Drawing for the job (mm, zero at the part's lowest x, y, z). A direction names the side the tool comes from. Round coordinates to 2 decimals unless told otherwise and drop trailing zeros. Write each loop counter-clockwise with the first axis right and the second up, starting at its lowest first coordinate (ties: lowest second). Pieces come first, ordered by that corner, then holes. Notation, with made-up numbers: (-19.5, 58) - (-5.5, 58) arc R30 cw to (-5.5, 87) - close; hole circle Ø7 at (-39.5, 34.25). An arc over 180 degrees is marked (long way). Answer in a Markdown table with one row per item.
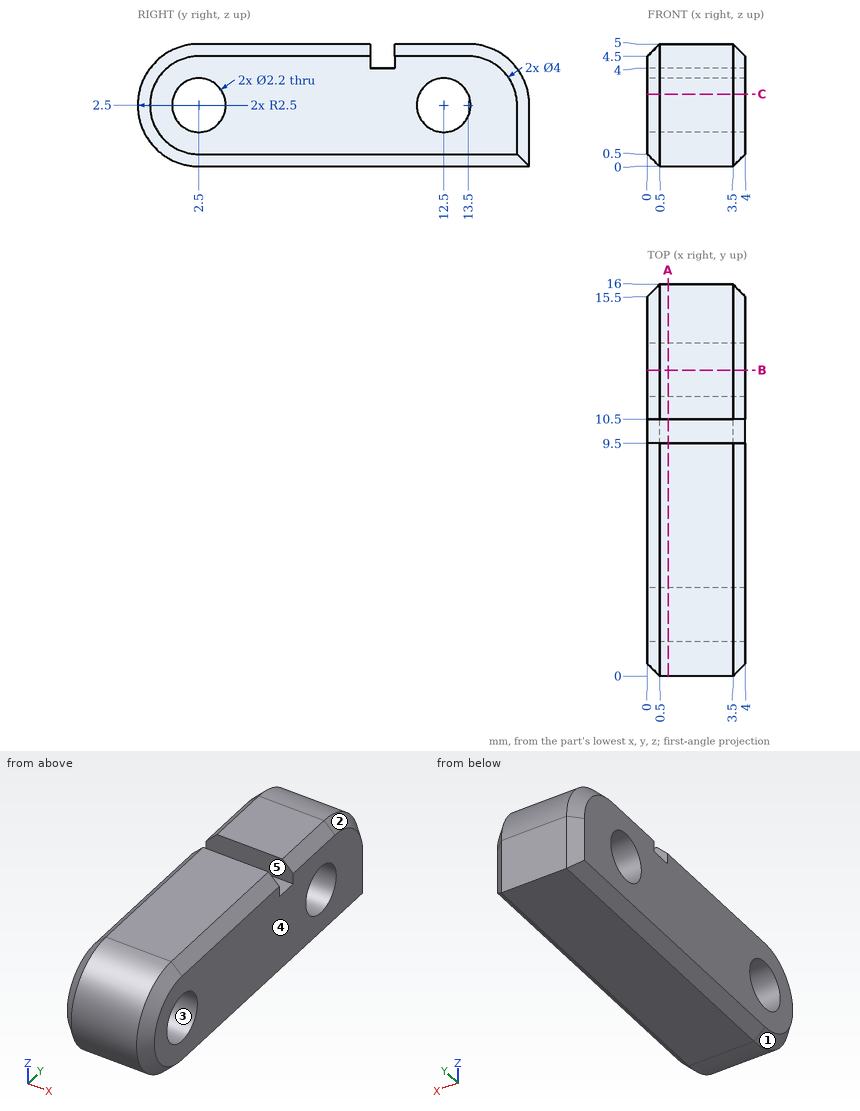
Q1. Flat gauge pins, fed straight in: pin 1 (1 mm diameter, centred on x = 1.5, z = 0.5, fed in from -Y); pin 2 (0.8 mm diameter, centred on x = 1.5, z = 4.5, fed in from -Y); pin 3 (2 mm diameter, centred on x = 2.5, y = 6, fed in from -Z); pin 4 (2 mm diameter, centred on y = 2.5, z = 2.5, fed in from +X). Where does each tip first touch, or does it go through?
Computed:
| item | result |
|---|---|
| pin 1 | stops at y = 0.5 |
| pin 2 | stops at y = 0.58 |
| pin 3 | stops at z = 0 |
| pin 4 | passes through |
Q2. Pull direction Y, two halves, no side cores. Call the marked faces 1, 2 and 3: released by +Y, released by -Y, zero draft, split by the parting line, or undercut.
Computed:
| item | result |
|---|---|
| face 1 | released by -Y |
| face 2 | released by +Y |
| face 3 | undercut |
Q3. 3-axis set-ups, long thin cutter, end or side, ignore diameter. For the marked faces 4 and 5: which of +Z, -Z, +X, -X, +Y, -Y reach the whole face in a straight line?
Computed:
| item | result |
|---|---|
| face 4 | +Z, -Z, +X, +Y, -Y |
| face 5 | +Z, +X, -X |
Q4. Saw through at B-B on y = 12.5. List the corners of the cut face in (x, z).
Computed:
| item | result |
|---|---|
| outline | (0, 0.5) - (0.5, 0) - (3.5, 0) - (4, 0.5) - (4, 1.4) - (0, 1.4) - close; (0, 3.6) - (4, 3.6) - (4, 4.5) - (3.5, 5) - (0.5, 5) - (0, 4.5) - close |
Q5. Drill centre lines: line 1 (Z direction, x = 1.25, y = 12.5); line 2 (Z direction, x = 2.4, y = 1); line 3 (Z direction, x = 1.6, y = 1.75). Where is each one in solid material? Low to high.
Computed:
| item | result |
|---|---|
| line 1 | z = 0 to 1.4, 3.6 to 5 |
| line 2 | z = 0.5 to 4.5 |
| line 3 | z = 0.12 to 1.7, 3.3 to 4.88 |
Q6. Saw through at A-A on x = 0.85. List the corners of the cut face in (y, z), then the cut area to 3 significant figures.
Computed:
| item | result |
|---|---|
| outline | (2.5, 0) - (16, 0) - (16, 2.5) arc R2.5 ccw to (13.5, 5) - (10.5, 5) - (10.5, 4) - (9.5, 4) - (9.5, 5) - (2.5, 5) arc R2.5 ccw to start; hole circle Ø2.2 at (2.5, 2.5); hole circle Ø2.2 at (12.5, 2.5) |
| area | 67.4 mm2 |
Q7. Saw through at C-C on z = 2.95. Count the separate pieces of the cut face and the enclosed holes in it, then the cut area to 3 significant figures.
Computed:
| item | result |
|---|---|
| separate pieces | 3 |
| enclosed holes | 0 |
| area | 47.1 mm2 |
